Read the model definition and answer for the solid it produces. Units are mm, in the model's axes. A direction names the side the tool comes from. Coordinates: 2 decimals unless noted, no trailing zeros. Write each loop counter-clockwise with the first axis right and the second up, starting at its lowest first coordinate (ties: lowest second). Pieces come first, ordered by that corner, then holes.
(1) Find the intervals of material crossed by probe 1 along Y at (x, z) = (6.5, 38.5); probe 2 along X at (y, z) = (-8.5, 70); probe 3 along Y at (x, z) = (-26.5, 9), in increasing order.
(2) Section A-A on z = 58 is taken. Write down the section's boundary in (x, y).
(3) The mould has two halves that part along Y. Classify faces 3 (the flat face through (-11, 11, 114.3)), 4 (the flat face through (0, -36.83, 58)), 5 (the flat face through (0, 36.83, 58)), 6 (the flat face through (-1, -38.1, 56)): +Y half, -Y half, draft (parallel to the pull), parting line (faces both ways), or undercut.
(4) Section C-C on x = 5 is taken. Write down the section's boundary in (y, z), then the cut area to 3 significant figures.
(5) Section B-B on y = 30.5 is taken. Write down the section's boundary in (x, z), then the cut area to 3 significant figures.
(6) Which of the six approach directions +Z, -Z, +X, -X, +Y, -Y give full straight-line access (tool end or side, diameter ignored) to faces 1 (the flat face through (-17, -16, 2.54)), 2 (the flat face through (-1, 1, 0))?
from build123d import *

# Parameters (mm, degrees)
F1_DEPTH = 2.54
F2_DEPTH = 114.3


with BuildPart() as f1:
    # F0 (on Top) → F1 (new body)
    with BuildSketch(Plane.XY):
        Polygon((35.9319743879, -36.83), (-36.83, 35.9319743879), (-36.83, -36.83), align=None)
    extrude(amount=F1_DEPTH)



with BuildPart() as f1b:
    # F0 (on Top) → F1, piece 2 (new body)
    with BuildSketch(Plane.XY):
        Polygon((36.83, 36.83), (-35.9319743879, 36.83), (36.83, -35.9319743879), align=None)
    extrude(amount=F1_DEPTH)


with BuildPart() as f1_1:
    add(f1.part)

    add(f1b.part)  # F2 merges F1b
    # F0 (on Top) → F2 (join)
    with BuildSketch(Plane.XY):
        with BuildLine():
            Line((-37.465, 38.1), (-38.1, 38.1))
            Line((-38.1, 38.1), (-38.1, 37.465))
            ThreePointArc((-38.1, 37.465), (-37.6509871939, 37.6509871939), (-37.465, 38.1))
        make_face()
        with BuildLine():
            Line((-37.2019743879, 38.1), (-37.465, 38.1))
            ThreePointArc((-37.465, 38.1), (-37.6509871939, 37.6509871939), (-38.1, 37.465))
            Line((-38.1, 37.465), (-38.1, 37.2019743879))
            Line((-38.1, 37.2019743879), (-36.83, 35.9319743879))
            Line((-36.83, 35.9319743879), (-36.83, 36.83))
            Line((-36.83, 36.83), (-35.9319743879, 36.83))
            Line((-35.9319743879, 36.83), (-37.2019743879, 38.1))
        make_face()
        Polygon((-36.83, 35.9319743879), (-38.1, 37.2019743879), (-38.1, -38.1), (37.2019743879, -38.1), (35.9319743879, -36.83), (-36.83, -36.83), align=None)
        Polygon((36.83, -35.9319743879), (-35.9319743879, 36.83), (-36.83, 36.83), (-36.83, 35.9319743879), (35.9319743879, -36.83), (36.83, -36.83), align=None)
        Polygon((38.1, 38.1), (-37.2019743879, 38.1), (-35.9319743879, 36.83), (36.83, 36.83), (36.83, -35.9319743879), (38.1, -37.2019743879), align=None)
        with BuildLine():
            Line((38.1, -37.465), (38.1, -37.2019743879))
            Line((38.1, -37.2019743879), (36.83, -35.9319743879))
            Line((36.83, -35.9319743879), (36.83, -36.83))
            Line((36.83, -36.83), (35.9319743879, -36.83))
            Line((35.9319743879, -36.83), (37.2019743879, -38.1))
            Line((37.2019743879, -38.1), (37.465, -38.1))
            ThreePointArc((37.465, -38.1), (37.6509871939, -37.6509871939), (38.1, -37.465))
        make_face()
        with BuildLine():
            Line((38.1, -38.1), (38.1, -37.465))
            ThreePointArc((38.1, -37.465), (37.6509871939, -37.6509871939), (37.465, -38.1))
            Line((37.465, -38.1), (38.1, -38.1))
        make_face()
    extrude(amount=F2_DEPTH)


solid = f1_1.part
Response:
1. probe 1: y = -38.1 to -36.83, -7.4 to -5.6, 36.83 to 38.1
1. probe 2: x = -38.1 to -36.83, 7.6 to 9.4, 36.83 to 38.1
1. probe 3: y = -38.1 to -36.83, 25.6 to 27.4, 36.83 to 38.1
2. outline: (-38.1, -38.1) - (38.1, -38.1) - (38.1, 38.1) - (-38.1, 38.1) - close; hole (-36.83, -36.83) - (35.93, -36.83) - (-36.83, 35.93) - close; hole (-35.93, 36.83) - (36.83, -35.93) - (36.83, 36.83) - close
3. face 3: draft
3. face 4: undercut
3. face 5: undercut
3. face 6: -Y half
4. outline: (-38.1, 0) - (38.1, 0) - (38.1, 114.3) - (36.83, 114.3) - (36.83, 2.54) - (-4.1, 2.54) - (-4.1, 114.3) - (-5.9, 114.3) - (-5.9, 2.54) - (-36.83, 2.54) - (-36.83, 114.3) - (-38.1, 114.3) - close
4. area: 678 mm2
5. outline: (-38.1, 0) - (38.1, 0) - (38.1, 114.3) - (36.83, 114.3) - (36.83, 2.54) - (-29.6, 2.54) - (-29.6, 114.3) - (-31.4, 114.3) - (-31.4, 2.54) - (-36.83, 2.54) - (-36.83, 114.3) - (-38.1, 114.3) - close
5. area: 678 mm2
6. face 1: +Z
6. face 2: -Z, +X, -X, +Y, -Y
